```python
from build123d import *

# Parameters (mm, degrees)
BOSS_EXTRUDE1_DEPTH = 30
BOSS_EXTRUDE1_TAPER = 4
BOSS_EXTRUDE2_DEPTH = 35
SKETCH5_W           = 10.352761804
SKETCH5_H           = 35
BOSS_EXTRUDE3_DEPTH = 27


with BuildPart() as part:
    # Sketch1 → Boss-Extrude1 (new body)
    with BuildSketch(Plane(origin=(0, 0, 0), x_dir=(1, 0, 0), z_dir=(0, 1, 0))):
        Polygon((-20, 0), (-17.320508076, -10), (-10, -17.320508076), (0, -20), (10, -17.320508076), (17.320508076, -10), (20, 0), (17.320508076, 10), (10, 17.320508076), (0, 20), (-10, 17.320508076), (-17.320508076, 10), align=None)
    extrude(amount=BOSS_EXTRUDE1_DEPTH, taper=BOSS_EXTRUDE1_TAPER)



with BuildPart() as body_2:
    # Sketch3 → Boss-Extrude2 (new body)
    with BuildSketch(Plane(origin=(0, 0, 0), x_dir=(-1, 0, 0), z_dir=(0, -1, 0))):
        with BuildLine():
            Line((10, -17.320508076), (0, -20))
            ThreePointArc((0, -20), (5.176380902, -19.318516526), (10, -17.320508076))
        make_face()
    extrude(amount=-BOSS_EXTRUDE2_DEPTH)


with BuildPart() as part_1:
    add(part.part)

    add(body_2.part)  # Boss-Extrude3 merges body 2
    # Sketch5 → Boss-Extrude3 (add)
    with BuildSketch(Plane(origin=(-5, 0, 18.660254038), x_dir=(-0.9659258262890708, 0, -0.2588190451025115), z_dir=(0.2588190451025115, 0, -0.9659258262890709))):
        with Locations((0, 17.5)):
            Rectangle(SKETCH5_W, SKETCH5_H)
    extrude(amount=BOSS_EXTRUDE3_DEPTH)


solid = part_1.part
```
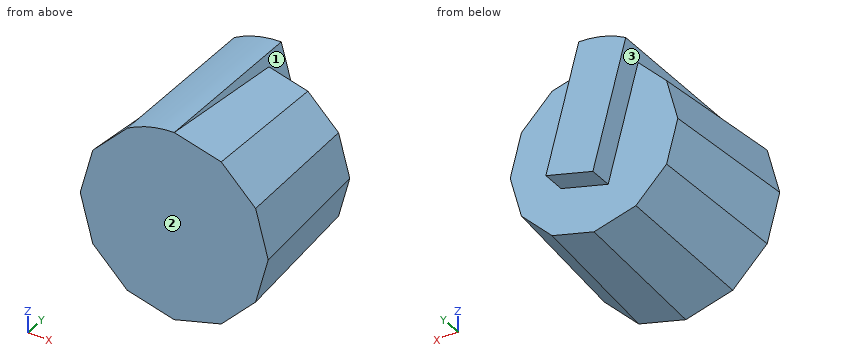
For this review, take the finished solid that the model builds, in its own axes (mm). Face numbers are marked on the shaded views. Round coordinates to 2 decimals unless told otherwise and drop trailing zeros. Write each loop counter-clockwise with the first axis right and the second up, starting at its lowest first coordinate (ties: lowest second). Pieces come first, ordered by that corner, then holes. Notation, with made-up numbers: M 41,-8 L 58,-8 A14 ccw 58,7 Z; hole C 82,88.25 d11. An arc over 180 degrees is marked long. One line per item, written item: value. Start each with the question number.
(1) Insertion check: pin 1 (1.5 mm diameter, centred on x = 12, z = 11, fed in from +Y); pin 2 (1.5 mm diameter, centred on y = 17.5, z = 8.5, fed in from +X); pin 3 (12 mm diameter, centred on x = -4.5, y = 6.5, fed in from -Z). Each pin has a flat end and moves straight along its axis. Give the tip position at first contact, or say it passes through.
(2) The part is to be moulded in two halves that separate along Z. For the marked faces 1, 2 and 3, say which applies: released by +Z, released by -Z, zero draft, split by the parting line, or undercut.
(3) We need section A-A (y = 32). Give the boundary of the cut face in (x, z), and give its area (3 significant figures).
(4) Wall thickness on line 1 (Y direction, x = -12, z = 5); line 2 (X direction, y = 21, z = -13); line 3 (X direction, y = 18.5, z = -0.5): over which ranges is each line inside the solid? List them lowest first.
Result:
1. pin 1: y = 30
1. pin 2: x = 16.66
1. pin 3: z = -19.82
2. face 1: released by +Z
2. face 2: zero draft
2. face 3: undercut
3. outline: M -10,17.32 L -3.01,-8.76 L 6.99,-6.08 L 0,20 A20 ccw Z
3. area: 284 mm²
4. line 1: 0 to 30
4. line 2: -12.24 to 12.24
4. line 3: -18.53 to 18.53
